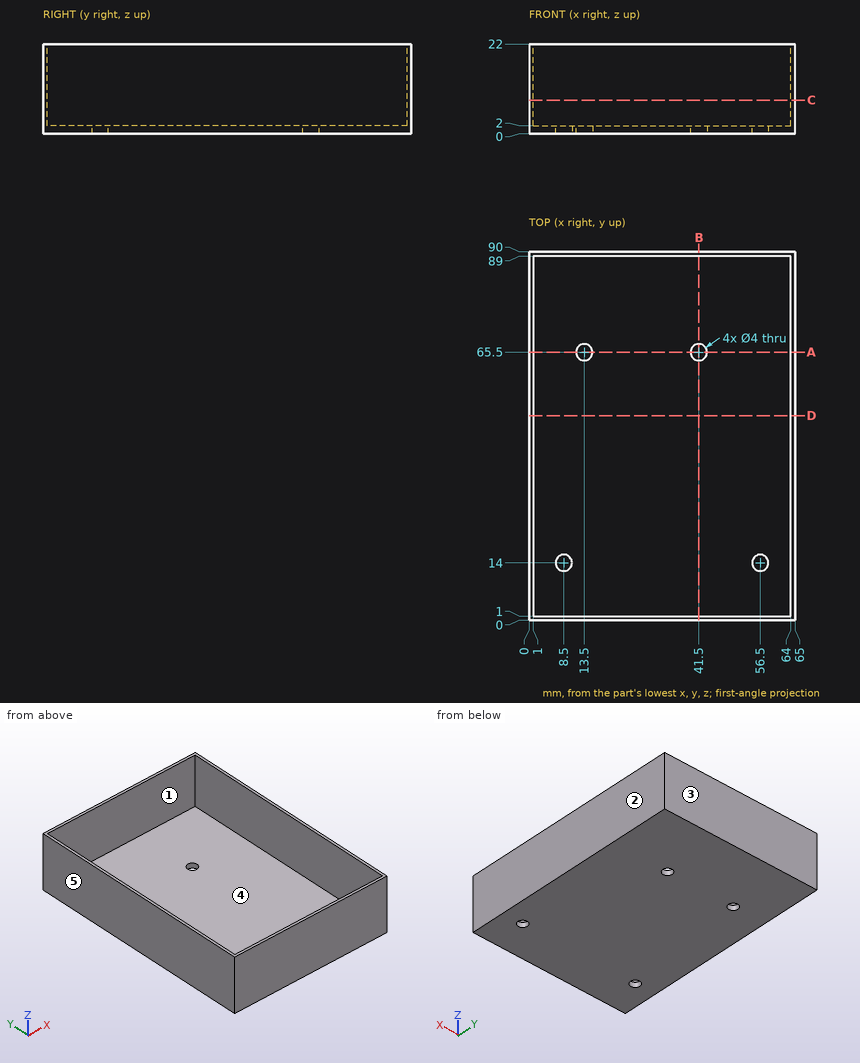
The drawing under review shows one solid part. Ordinate dimensions are in mm from its lowest x, y, z. A direction names the side the tool comes from. Coordinates: 2 decimals unless noted, no trailing zeros. Order: outer loops, then holes, each group sorted by start corner. A loop starts at its lowest first (then second) coordinate and runs counter-clockwise, first axis right, second up. Notation, with made-up numbers: (-21, 27) - (6, 27) arc R18 ccw to (6, 55) - close; hole circle Ø2 at (-22.75, 37.25). An arc over 180 degrees is marked (long way). Put each result on its own line as item: value.
1) Tool access review of the marked faces 4 and 5: name each direction out of +Z, -Z, +X, -X, +Y, -Y from which nothing blocks a thin tool from reaching the whole face with its end or side.
Response values:
face 4: +Z
face 5: +Z, -Z, -X, +Y, -Y
2) Take a section at A-A, the plane y = 65.5. Give the boundary of the cut face in (x, z).
Response values:
outline: (0, 0) - (11.5, 0) - (11.5, 2) - (1, 2) - (1, 22) - (0, 22) - close; (15.5, 0) - (39.5, 0) - (39.5, 2) - (15.5, 2) - close; (43.5, 0) - (65, 0) - (65, 22) - (64, 22) - (64, 2) - (43.5, 2) - close
3) Insertion check: P1, Ø4, axis at x = 55.5, y = 12, coming from the +Z side. The pin has a flat end and moves straight along its axis. Give the tip position at first contact, or say it passes through.
Response values:
P1: stops at z = 2
4) Take a section at B-B, the plane x = 41.5. Give the boundary of the cut face in (y, z), and give its area (3 significant figures).
Response values:
outline: (0, 0) - (63.5, 0) - (63.5, 2) - (1, 2) - (1, 22) - (0, 22) - close; (67.5, 0) - (90, 0) - (90, 22) - (89, 22) - (89, 2) - (67.5, 2) - close
area: 212 mm²
5) Take a section at C-C, the plane z = 8.25. Give the boundary of the cut face in (x, y), and give its area (3 significant figures).
Response values:
outline: (0, 0) - (65, 0) - (65, 90) - (0, 90) - close; hole (1, 1) - (64, 1) - (64, 89) - (1, 89) - close
area: 306 mm²
6) The part is to be moulded in two halves that separate along Y. For the marked faces 1, 2 and 3, say which applies: released by +Y, released by -Y, zero draft, split by the parting line, or undercut.
Response values:
face 1: undercut
face 2: zero draft
face 3: released by +Y
7) Take a section at D-D, the plane y = 50. Give the boundary of the cut face in (x, z).
Response values:
outline: (0, 0) - (65, 0) - (65, 22) - (64, 22) - (64, 2) - (1, 2) - (1, 22) - (0, 22) - close
8) Wall thickness on L1, parallel to Y at x = 55.5, z = 2.5; L2, parallel to X at y = 31.5, z = 19.75; L3, parallel to Y at x = 56.5, z = 1.1: over which ranges is each line inside the solid? List them lowest first. Write a range as from..to.
Response values:
L1: y = 0..1, 89..90
L2: x = 0..1, 64..65
L3: y = 0..12, 16..90
